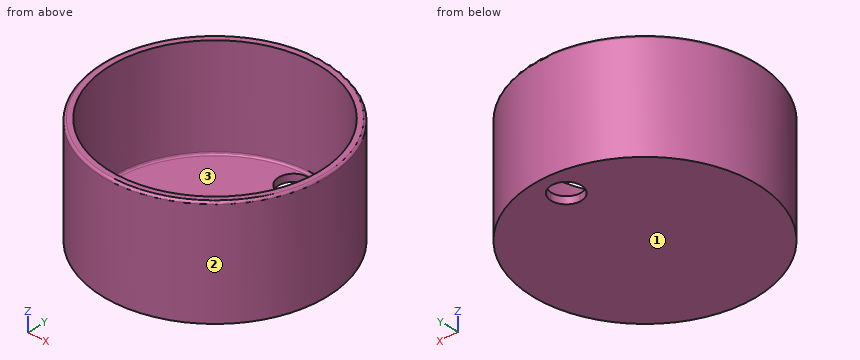
```python
from build123d import *

# Parameters (mm, degrees)
F0_R     = 39.497
F1_DEPTH = 38.1
F2_R     = 36.957
F3_DEPTH = 35.56
F4_R     = 0.762
F5_R     = 0.762
F7_DEPTH = 25.4


with BuildPart() as f1:
    # F0 (on Top) → F1 (new body)
    with BuildSketch(Plane.XY):
        Circle(F0_R)
    extrude(amount=F1_DEPTH)

    # F2 (on face) → F3 (cut)
    with BuildSketch(Plane.XY.offset(38.1)):
        Circle(F2_R)
    extrude(amount=-F3_DEPTH, mode=Mode.SUBTRACT)

    # F4
    f4_edges = [f1.edges().sort_by_distance(p)[0] for p in [
        (-36.957, 0, 2.54),
    ]]
    fillet(f4_edges, radius=F4_R)

    # F5
    f5_edges = [f1.edges().sort_by_distance(p)[0] for p in [
        (-39.497, 0, 38.1),
    ]]
    fillet(f5_edges, radius=F5_R)

    # F6 (on face) → F7 (cut)
    with BuildSketch(Plane(origin=(0, 0, 0), x_dir=(1, 0, 0), z_dir=(0, 0, -1))):
        with BuildLine():
            Line((0, -25.019), (0, -30.353))
            Line((0, -30.353), (0, -35.687))
            ThreePointArc((0, -35.687), (3.771708, -34.124708), (5.334, -30.353))
            ThreePointArc((5.334, -30.353), (3.771708, -26.581292), (0, -25.019))
        make_face()
        with BuildLine():
            Line((0, -35.687), (0, -30.353))
            Line((0, -30.353), (0, -25.019))
            ThreePointArc((0, -25.019), (-5.334, -30.353), (0, -35.687))
        make_face()
    extrude(amount=-F7_DEPTH, mode=Mode.SUBTRACT)


solid = f1.part
```
For this review, take the finished solid that the model builds, in its own axes (mm). Face numbers are marked on the shaded views. Give positions to 0.01 mm unless a question says otherwise; leave off trailing zeros. Write each loop counter-clockwise with the first axis right and the second up, starting at its lowest first coordinate (ties: lowest second). Pieces come first, ordered by that corner, then holes.
Item 1: Wall thickness on probe 1 along Y at (x, z) = (0, 20); probe 2 along Z at (x, y) = (0.5, -32.5); probe 3 along X at (y, z) = (-34, 9): over which ranges is each line inside the solid? List them lowest first.
Item 2: Take a section at B-B (z = 27.5). Give the boundary of the cut face in (x, y), and give its area (3 significant figures).
Item 3: Insertion check: P1, Ø1, axis at y = 16, z = 30.5, coming from the -X side; P2, Ø4, axis at x = 22.5, z = 19, coming from the +Y side; P3, Ø2, axis at x = 18.5, z = 13, coming from the +Y side. Each pin has a flat end and moves straight along its axis. Give the tip position at first contact, or say it passes through.
Item 4: The part is to be moulded in two halves that separate along X. For the marked faces 1, 2 and 3, say which applies: +X half, -X half, draft (parallel to the pull), parting line (faces both ways), or undercut.
Item 5: Take a section at A-A (y = 0). Give the boundary of the cut face in (x, z) (3 decimals), and give its area (3 significant figures).
Established:
1. probe 1: y = -39.5 to -36.96, 36.96 to 39.5
1. probe 2: z = 0 to 2.54
1. probe 3: x = -20.1 to -14.49, 14.49 to 20.1
2. outline: circle Ø78.99 at (0, 0); hole circle Ø73.91 at (0, 0)
2. area: 610 mm2
3. P1: stops at x = -36.33
3. P2: stops at y = 33.76
3. P3: stops at y = 35.41
4. face 1: draft
4. face 2: parting line
4. face 3: undercut
5. outline: (-39.497, 0) - (39.497, 0) - (39.497, 37.338) arc R0.762 ccw to (38.735, 38.1) - (36.957, 38.1) - (36.957, 3.302) arc R0.762 cw to (36.195, 2.54) - (-36.195, 2.54) arc R0.762 cw to (-36.957, 3.302) - (-36.957, 38.1) - (-38.735, 38.1) arc R0.762 ccw to (-39.497, 37.338) - close
5. area: 381 mm2
